```python
from build123d import *

# Parameters (mm, degrees)
SKETCH2_W           = 45
SKETCH2_H           = 10
BOSS_EXTRUDE1_DEPTH = 40
SKETCH4_W           = 45
SKETCH4_H           = 10
BOSS_EXTRUDE2_DEPTH = 10
SKETCH8_W           = 45
SKETCH8_H           = 10
BOSS_EXTRUDE3_DEPTH = 20
SKETCH9_R           = 1.45
CUT_EXTRUDE2_DEPTH  = 20
SKETCH10_W          = 45
SKETCH10_H          = 0.626165357
CUT_EXTRUDE3_DEPTH  = 2
SKETCH11_W          = 19
SKETCH11_H          = 42.671327575
BOSS_EXTRUDE4_DEPTH = 1.5
SKETCH12_W          = 3
SKETCH12_H          = 27.286335608
CUT_EXTRUDE6_DEPTH  = 10


with BuildPart() as part:
    # Sketch2 → Boss-Extrude1 (new body)
    with BuildSketch(Plane(origin=(0, 0, 0), x_dir=(1, 0, 0), z_dir=(0, 1, 0))):
        Rectangle(SKETCH2_W, SKETCH2_H)
    extrude(amount=BOSS_EXTRUDE1_DEPTH)

    # Sketch4 → Boss-Extrude2 (add)
    with BuildSketch(Plane(origin=(0, 40, 0), x_dir=(1, 0, 0), z_dir=(0, 1, 0))):
        Rectangle(SKETCH4_W, SKETCH4_H)
    extrude(amount=BOSS_EXTRUDE2_DEPTH)

    # Sketch8 → Boss-Extrude3 (add)
    with BuildSketch(Plane.XZ):
        Rectangle(SKETCH8_W, SKETCH8_H)
    extrude(amount=BOSS_EXTRUDE3_DEPTH)

    # Sketch9 → Cut-Extrude2 (cut)
    with BuildSketch(Plane.XY.offset(5)):
        with Locations((19.5, 11.5)):
            Circle(SKETCH9_R)
        with Locations((-19.5, 11.5)):
            Circle(SKETCH9_R)
    extrude(amount=-CUT_EXTRUDE2_DEPTH, mode=Mode.SUBTRACT)

    # Sketch10 → Cut-Extrude3 (cut)
    with BuildSketch(Plane.XY.offset(5)):
        with Locations((0, 22.984410254)):
            Rectangle(SKETCH10_W, SKETCH10_H)
    extrude(amount=-CUT_EXTRUDE3_DEPTH, mode=Mode.SUBTRACT)

    # Sketch11 → Boss-Extrude4 (add)
    with BuildSketch(Plane.XY.offset(5)):
        with Locations((0, 1.335663788)):
            Rectangle(SKETCH11_W, SKETCH11_H)
    extrude(amount=BOSS_EXTRUDE4_DEPTH)

    # Sketch12 → Cut-Extrude6 (cut)
    with BuildSketch(Plane(origin=(22.5, 0, 0), x_dir=(0, 0, -1), z_dir=(1, 0, 0))):
        with Locations((0, -4.971840229)):
            Rectangle(SKETCH12_W, SKETCH12_H)
    extrude(amount=-CUT_EXTRUDE6_DEPTH, mode=Mode.SUBTRACT)


solid = part.part
```
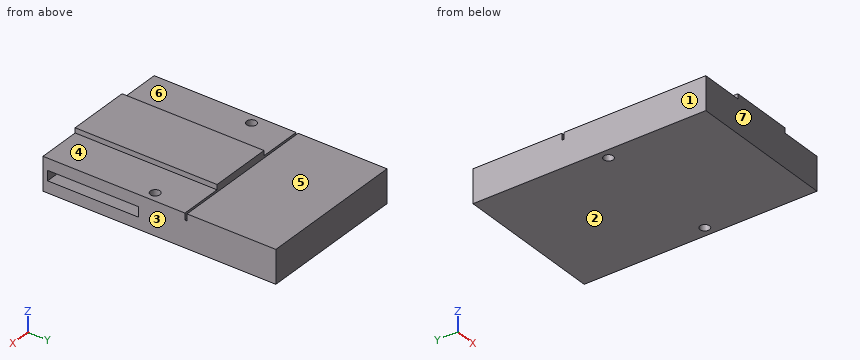
Part model, mm, in its own coordinate system. Face numbers are marked on the shaded views. A direction names the side the tool comes from. Coordinates: 2 decimals unless noted, no trailing zeros. Write each loop counter-clockwise with the first axis right and the second up, starting at its lowest first coordinate (ties: lowest second). Pieces come first, ordered by that corner, then holes.
Item 1: Slice it at A-A (x = -19.5). Write the cut outline in (y, z).
Item 2: Probe line 1 (Y direction, x = 20.5, z = 1) (3 decimals); line 2 (Y direction, x = 20, z = -0.5) (3 decimals); line 3 (Z direction, x = 10, y = -11.5). List the from-to ranges inside material, lowest first.
Item 3: Mould opens along X. For the marked faces 1, 2 and 3 say: released by +X, released by -X, zero draft, split by the parting line, or undercut.
Item 4: Pin check, flat tips, straight feed: pin 1 (1.7 mm diameter, centred on x = 19.5, y = 11.5, fed in from -Z); pin 2 (10.5 mm diameter, centred on x = -19, y = -4, fed in from +Z); pin 3 (0.8 mm diameter, centred on y = -3.5, z = 5.5, fed in from +X); pin 4 (0.5 mm diameter, centred on x = 3, y = 23, fed in from +Z). Stop position of each tip, or through.
Item 5: Slice it at C-C (y = 11.5). Write the cut outline in (x, z), and give its area (4 significant figures).
Item 6: Slice it at B-B (x = 19.5). Count the separate pieces of the cut face and the enclosed holes in it, and give its area (3 significant figures).
Item 7: Which spindle directions (+Z, -Z, +X, -X, +Y, -Y) get a long thin tool onto all of the face, cutting with end or side? Do the marked faces 4, 5, 6 and 7. Say none if no direction does.
Item 8: Slice it at D-D (x = 3). Write the cut outline in (y, z).
Results found:
1. outline: (-20, -5) - (10.05, -5) - (10.05, 5) - (-20, 5) - close; (12.95, -5) - (50, -5) - (50, 5) - (23.3, 5) - (23.3, 3) - (22.67, 3) - (22.67, 5) - (12.95, 5) - close
2. line 1: y = -20 to -18.615, 8.671 to 10.45, 12.55 to 50
2. line 2: y = -20 to -18.615, 8.671 to 10.139, 12.861 to 50
2. line 3: z = -5 to 5
3. face 1: released by -X
3. face 2: zero draft
3. face 3: released by +X
4. pin 1: passes through
4. pin 2: stops at z = 5
4. pin 3: stops at x = 9.5
4. pin 4: stops at z = 3
5. outline: (-22.5, -5) - (-20.95, -5) - (-20.95, 5) - (-22.5, 5) - close; (-18.05, -5) - (18.05, -5) - (18.05, 5) - (9.5, 5) - (9.5, 6.5) - (-9.5, 6.5) - (-9.5, 5) - (-18.05, 5) - close; (20.95, -5) - (22.5, -5) - (22.5, 5) - (20.95, 5) - close
5. area: 420.5 mm2
6. separate pieces: 2
6. enclosed holes: 1
6. area: 588 mm2
7. face 4: +Z, +X, +Y, -Y
7. face 5: +Z, +X, -X, +Y
7. face 6: +Z, -X, +Y, -Y
7. face 7: +Z, -Z, +X, -X, -Y
8. outline: (-20, -5) - (50, -5) - (50, 5) - (23.3, 5) - (23.3, 3) - (22.67, 3) - (22.67, 6.5) - (-20, 6.5) - close
